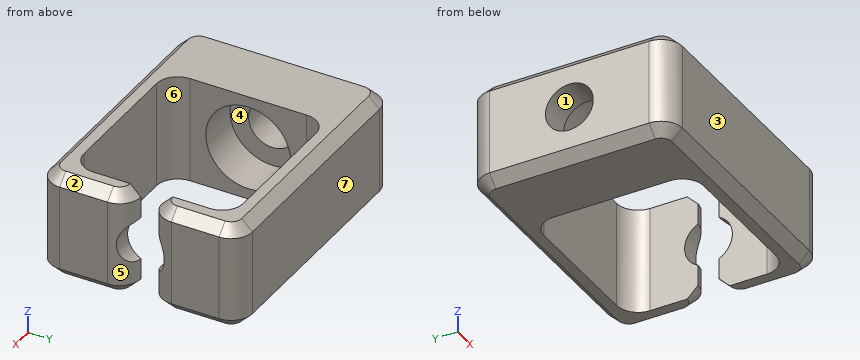
from build123d import *

# Parameters (mm, degrees)
F1_DEPTH    = 5
F2_R        = 2.25
F3_DEPTH    = 100
F4_R        = 4
F5_DEPTH    = 4
F6_T1_DEPTH = 10
F6_T3_DEPTH = 20
F6_T5_DEPTH = 12.9844355629
F6_T7_DEPTH = 12.9844355629
F7_SIZE     = 1


# Not quite as in the source:
# - a fillet or chamfer that OpenCascade refuses, or shapes differently, is made with other operations: its cross-section is extruded or revolved along the edge and cut away or added


with BuildPart() as f1:
    # F0 (on Top) → F1 (new body, symmetric)
    with BuildSketch(Plane.XY):
        Polygon((12.5, 1), (12.5, 9.5), (-12.5, 9.5), (-12.5, -9.5), (12.5, -9.5), (12.5, -1), (10.5, -1), (10.5, -7.5), (-5.5, -7.5), (-5.5, 7.5), (10.5, 7.5), (10.5, 1), align=None)
    extrude(amount=F1_DEPTH, both=True)

    # F2 (on face) → F3 (cut, symmetric)
    with BuildSketch(Plane.YZ.offset(-5.5)):
        Circle(F2_R)
    extrude(amount=F3_DEPTH, both=True, mode=Mode.SUBTRACT)

    # F4 (on face) → F5 (cut)
    with BuildSketch(Plane.YZ.offset(-5.5)):
        Circle(F4_R)
    extrude(amount=-F5_DEPTH, mode=Mode.SUBTRACT)

    # F6: fillet of radius 2 on 12 edges, made by hand

    # F6_s2 → F6_t1 (join)
    with BuildSketch(Plane.XY.offset(-5)):
        with BuildLine():
            ThreePointArc((10.5, -5.5), (9.9142135624, -6.9142135624), (8.5, -7.5))
            Line((8.5, -7.5), (10.5, -7.5))
            Line((10.5, -7.5), (10.5, -5.5))
        make_face()
        with BuildLine():
            ThreePointArc((10.5, 5.5), (9.9142135624, 6.9142135624), (8.5, 7.5))
            Line((8.5, 7.5), (10.5, 7.5))
            Line((10.5, 7.5), (10.5, 5.5))
        make_face()
        with BuildLine():
            ThreePointArc((-5.5, 5.5), (-4.9142135624, 6.9142135624), (-3.5, 7.5))
            Line((-3.5, 7.5), (-5.5, 7.5))
            Line((-5.5, 7.5), (-5.5, 5.5))
        make_face()
        with BuildLine():
            ThreePointArc((-3.5, -7.5), (-4.9142135624, -6.9142135624), (-5.5, -5.5))
            Line((-5.5, -5.5), (-5.5, -7.5))
            Line((-5.5, -7.5), (-3.5, -7.5))
        make_face()
    extrude(amount=F6_T1_DEPTH)

    # F6_s4 → F6_t3 (cut)
    with BuildSketch(Plane.XY.offset(-10)):
        with BuildLine():
            ThreePointArc((-10.5, 9.5), (-11.9142135624, 8.9142135624), (-12.5, 7.5))
            Line((-12.5, 7.5), (-12.5, 9.5))
            Line((-12.5, 9.5), (-10.5, 9.5))
        make_face()
        with BuildLine():
            ThreePointArc((-12.5, -7.5), (-11.9142135624, -8.9142135624), (-10.5, -9.5))
            Line((-10.5, -9.5), (-12.5, -9.5))
            Line((-12.5, -9.5), (-12.5, -7.5))
        make_face()
        with BuildLine():
            ThreePointArc((12.5, 7.5), (11.9142135624, 8.9142135624), (10.5, 9.5))
            Line((10.5, 9.5), (12.5, 9.5))
            Line((12.5, 9.5), (12.5, 7.5))
        make_face()
        with BuildLine():
            ThreePointArc((10.5, -9.5), (11.9142135624, -8.9142135624), (12.5, -7.5))
            Line((12.5, -7.5), (12.5, -9.5))
            Line((12.5, -9.5), (10.5, -9.5))
        make_face()
    extrude(amount=F6_T3_DEPTH, mode=Mode.SUBTRACT)

    # F6_s6 → F6_t5 (cut)
    with BuildSketch(Plane.XY.offset(-2.9844355629)):
        with BuildLine():
            ThreePointArc((12.5, -3), (11.9142135624, -1.5857864376), (10.5, -1))
            Line((10.5, -1), (12.5, -1))
            Line((12.5, -1), (12.5, -3))
        make_face()
        with BuildLine():
            ThreePointArc((12.5, 3), (11.9142135624, 1.5857864376), (10.5, 1))
            Line((10.5, 1), (12.5, 1))
            Line((12.5, 1), (12.5, 3))
        make_face()
    extrude(amount=F6_T5_DEPTH, mode=Mode.SUBTRACT)

    # F6_s8 → F6_t7 (cut)
    with BuildSketch(Plane.XY.offset(-10)):
        with BuildLine():
            ThreePointArc((12.5, -3), (11.9142135624, -1.5857864376), (10.5, -1))
            Line((10.5, -1), (12.5, -1))
            Line((12.5, -1), (12.5, -3))
        make_face()
        with BuildLine():
            ThreePointArc((12.5, 3), (11.9142135624, 1.5857864376), (10.5, 1))
            Line((10.5, 1), (12.5, 1))
            Line((12.5, 1), (12.5, 3))
        make_face()
    extrude(amount=F6_T7_DEPTH, mode=Mode.SUBTRACT)

    # F7
    f7_edges = [f1.edges().sort_by_distance(p)[0] for p in [
        (0, 9.5, 5),
        (-12.5, 0, -5),
    ]]
    chamfer(f7_edges, length=F7_SIZE)


solid = f1.part
CAD build for the part. Positions are in the model's coordinates, mm. Face numbers are marked on the shaded views. A direction names the side the tool comes from. Give positions to 0.01 mm unless a question says otherwise; leave off trailing zeros. Loops run counter-clockwise (first coordinate to the right, second up) from the corner with the lowest first, then second, coordinate; pieces in that order, holes last. Notation, with made-up numbers: M 66,46 L 81,46 A28 ccw 81,66 Z; hole C -3.75,16 d1. An arc over 180 degrees is marked long. Write each question's results on one line, items separated by ' | '.
Q1. Band-saw the part on B-B on x = 8. Write the cut outline in (y, z).
Geometry check:
outline: M -9.5,-4 L -8.5,-5 L -7.5,-5 L -7.5,5 L -8.5,5 L -9.5,4 Z; M 7.5,-5 L 8.5,-5 L 9.5,-4 L 9.5,4 L 8.5,5 L 7.5,5 Z
Q2. Band-saw the part on A-A on y = 0. Write the cut outline in (x, z), and give its area (3 significant figures).
Geometry check:
outline: M -12.5,-4 L -11.5,-5 L -5.5,-5 L -5.5,-4 L -9.5,-4 L -9.5,-2.25 L -12.5,-2.25 Z; M -12.5,2.25 L -9.5,2.25 L -9.5,4 L -5.5,4 L -5.5,5 L -11.5,5 L -12.5,4 Z | area: 23.5 mm²
Q3. Which spindle directions (+Z, -Z, +X, -X, +Y, -Y) get a long thin tool onto all of the face, cutting with end or side? Do the marked faces 5, 6 and 7. Say none if no direction does.
Geometry check:
face 5: +Z, -Z, +X | face 6: +Z, -Z | face 7: +Z, -Z, +X, -X, +Y
Q4. Band-saw the part on D-D on y = -6.75. Write the cut outline in (x, z), and give its area (3 significant figures).
Geometry check:
outline: M -12.5,-4 L -11.5,-5 L -5.06,-5 L -5.06,5 L -11.5,5 L -12.5,4 Z; M 10.06,-5 L 11.5,-5 L 12.5,-4 L 12.5,4 L 11.5,5 L 10.06,5 Z | area: 96.8 mm²
Q5. Flat gauge pins, fed straight in: P1, Ø4, axis at y = -0.5, z = 0.5, coming from the +X side; P2, Ø3, axis at y = 0, z = 1.5, coming from the +X side; P3, Ø6, axis at x = -2.5, y = 6, coming from the +Z side; P4, Ø1.5, axis at x = 9, y = -1.5, coming from the +Z side. Where does each tip first touch, or does it go through?
Geometry check:
P1: stops at x = 12.44 | P2: stops at x = 11.81 | P3: stops at z = 5 | P4: passes through
Q6. Probe probe 1 along Y at (x, z) = (0.75, 2.5); probe 2 along Z at (x, y) = (-6.75, 0); probe 3 along X at (y, z) = (-4.25, 2.75). List the from-to ranges inside material, lowest first.
Geometry check:
probe 1: y = -9.5 to -7.5, 7.5 to 9.5 | probe 2: z = -5 to -4, 4 to 5 | probe 3: x = -12.5 to -5.5, 10.5 to 12.5
Q7. Mould opens along Z. For the marked faces 1, 2, 3 and 4 say: pulls with the +Z half, pulls with the -Z half, needs draft (parallel to the pull), parting line crosses it, or undercut.
Geometry check:
face 1: undercut | face 2: pulls with the +Z half | face 3: needs draft | face 4: undercut
